Part model, mm, in its own coordinate system. Round coordinates to 2 decimals unless told otherwise and drop trailing zeros. Write each loop counter-clockwise with the first axis right and the second up, starting at its lowest first coordinate (ties: lowest second). Pieces come first, ordered by that corner, then holes.
1) Saw through at D-D on x = 8. Write the cut outline in (y, z).
2) Drill centre lines: L1, parallel to Y at x = 6.25, z = -0.1; L2, parallel to Y at x = 4.5, z = 0.05; L3, parallel to Y at x = 2.75, z = 0.1. Where is each one in solid material? Low to high.
3) Saw through at B-B on z = 0.05. Write the cut outline in (x, y) (1 decimal).
4) Saw through at A-A on x = 7. Write the cut outline in (y, z).
5) Saw through at C-C on y = 1.5. Write the cut outline in (x, z).
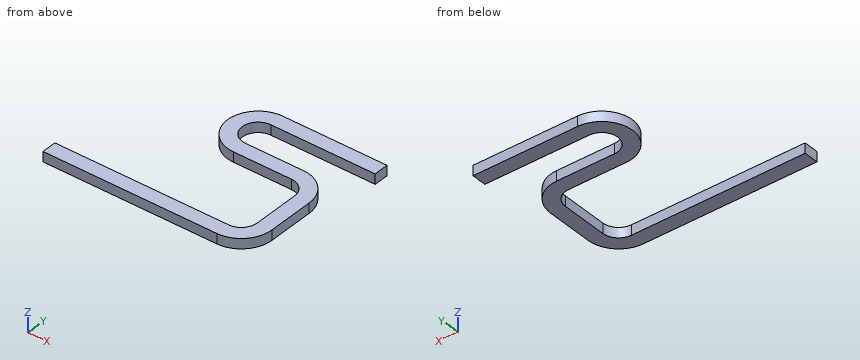
```python
from build123d import *

# Parameters (mm, degrees)
SKETCH2_W = 0.432
SKETCH2_H = 0.635


with BuildPart() as part:
    # Sweep1: sweep along a path in Sketch1
    with BuildLine(Plane.XY) as sweep1_path:
        Line((0, 0), (7.5, 0))
        ThreePointArc((7.5, 0), (8.207106781, 0.292893219), (8.5, 1))
        Line((8.5, 1), (8.5, 3))
        ThreePointArc((8.5, 3), (8.207106781, 3.707106781), (7.5, 4))
        Line((7.5, 4), (5, 4))
        ThreePointArc((5, 4), (4, 5), (5, 6))
        Line((5, 6), (9.5, 6))
    # Sketch2 → Sweep1 (sweep)
    with BuildSketch(Plane(origin=(0, 0, 0), x_dir=(0, 0, -1), z_dir=(1, 0, 0))):
        Rectangle(SKETCH2_W, SKETCH2_H)
    sweep(path=sweep1_path.line)


solid = part.part
```
Completed:
1. outline: (-0.22, -0.22) - (0.54, -0.22) - (0.54, 0.22) - (-0.22, 0.22) - close; (3.46, -0.22) - (4.22, -0.22) - (4.22, 0.22) - (3.46, 0.22) - close; (5.68, -0.22) - (6.32, -0.22) - (6.32, 0.22) - (5.68, 0.22) - close
2. L1: y = -0.32 to 0.32, 3.68 to 4.32, 5.68 to 6.32
2. L2: y = -0.32 to 0.32, 3.78 to 4.54, 5.46 to 6.22
2. L3: y = -0.32 to 0.32
3. outline: (0, -0.3) - (7.5, -0.3) arc R1.3 ccw to (8.8, 1) - (8.8, 3) arc R1.3 ccw to (7.5, 4.3) - (5, 4.3) arc R0.7 cw to (5, 5.7) - (9.5, 5.7) - (9.5, 6.3) - (5, 6.3) arc R1.3 ccw to (5, 3.7) - (7.5, 3.7) arc R0.7 cw to (8.2, 3) - (8.2, 1) arc R0.7 cw to (7.5, 0.3) - (0, 0.3) - close
4. outline: (-0.32, -0.22) - (0.32, -0.22) - (0.32, 0.22) - (-0.32, 0.22) - close; (3.68, -0.22) - (4.32, -0.22) - (4.32, 0.22) - (3.68, 0.22) - close; (5.68, -0.22) - (6.32, -0.22) - (6.32, 0.22) - (5.68, 0.22) - close
5. outline: (8.18, -0.22) - (8.82, -0.22) - (8.82, 0.22) - (8.18, 0.22) - close
